Read the model definition and answer for the solid it produces. Units are mm, in the model's axes. A direction names the side the tool comes from. Round coordinates to 2 decimals unless told otherwise and drop trailing zeros. Loops run counter-clockwise (first coordinate to the right, second up) from the corner with the lowest first, then second, coordinate; pieces in that order, holes last. Notation, with made-up numbers: M 22,32 L 45,32 A20 ccw 45,57 Z; hole C -21,61.25 d10. An arc over 180 degrees is marked long. Write each question's results on one line, items separated by ' | '.
from build123d import *

# Parameters (mm, degrees)
BOSS_EXTRUDE3_DEPTH                                 = 48
SKETCH9_R                                           = 1.6
BOSS_EXTRUDE5_DEPTH                                 = 2
SKETCH6_R                                           = 1.6
BOSS_EXTRUDE6_DEPTH                                 = 2
FILLET4_R                                           = 1
FILLET5_R                                           = 12.2
CSK_FOR_M3_COUNTERSUNK_FLAT_HEAD_SCREW1_D           = 3.2
CSK_FOR_M3_COUNTERSUNK_FLAT_HEAD_SCREW1_CSINK_D     = 6.3
CSK_FOR_M3_COUNTERSUNK_FLAT_HEAD_SCREW1_CSINK_ANGLE = 90
CSK_FOR_M3_COUNTERSUNK_FLAT_HEAD_SCREW2_D           = 3.2
CSK_FOR_M3_COUNTERSUNK_FLAT_HEAD_SCREW2_CSINK_D     = 6.3
CSK_FOR_M3_COUNTERSUNK_FLAT_HEAD_SCREW2_CSINK_ANGLE = 90


with BuildPart() as part:
    # Sketch5 → Boss-Extrude3 (new, symmetric)
    with BuildSketch(Plane(origin=(0, 0, 0), x_dir=(1, 0, 0), z_dir=(0, 1, 0))):
        Polygon((0, 8.5), (0, 0), (8.5, 0), (8.5, 2), (2, 2), (2, 8.5), align=None)
    extrude(amount=BOSS_EXTRUDE3_DEPTH, both=True)

    # Sketch9 → Boss-Extrude5 (add)
    with BuildSketch(Plane.XY):
        with BuildLine():
            Line((8.5, 50), (18.5, 50))
            Line((18.5, 50), (18.5, 48.8))
            Line((18.5, 48.8), (22.7, 48.8))
            Line((22.7, 48.8), (22.7, 44))
            ThreePointArc((22.7, 44), (21.821320344, 41.878679656), (19.7, 41))
            Line((19.7, 41), (8.5, 41))
            Line((8.5, 41), (8.5, 50))
        make_face()
        with Locations((11.9, 45.8)):
            Circle(SKETCH9_R, mode=Mode.SUBTRACT)
        with Locations((19.5, 45.8)):
            Circle(SKETCH9_R, mode=Mode.SUBTRACT)
    boss_extrude5 = extrude(amount=-BOSS_EXTRUDE5_DEPTH)

    # Sketch6 → Boss-Extrude6 (add)
    with BuildSketch(Plane.ZY):
        with BuildLine():
            Line((-8.5, 41), (-19.7, 41))
            ThreePointArc((-19.7, 41), (-21.821320344, 41.878679656), (-22.7, 44))
            Line((-22.7, 44), (-22.7, 48.8))
            Line((-22.7, 48.8), (-18.5, 48.8))
            Line((-18.5, 48.8), (-18.5, 50))
            Line((-18.5, 50), (-8.5, 50))
            Line((-8.5, 50), (-8.5, 41))
        make_face()
        with Locations((-11.9, 45.8)):
            Circle(SKETCH6_R, mode=Mode.SUBTRACT)
        with Locations((-19.5, 45.8)):
            Circle(SKETCH6_R, mode=Mode.SUBTRACT)
    boss_extrude6 = extrude(amount=-BOSS_EXTRUDE6_DEPTH)

    # Mirror1: Boss-Extrude5, Boss-Extrude6 across plane
    add(boss_extrude5.mirror(Plane.ZX))
    add(boss_extrude6.mirror(Plane.ZX))

    # Fillet4
    fillet4_edges = [part.edges().sort_by_distance(p)[0] for p in [
        (0, 0, 0),
        (13.5, 50, 0),
        (0, 50, -13.5),
    ]]
    fillet(fillet4_edges, radius=FILLET4_R)

    # Fillet5
    fillet5_edges = [part.edges().sort_by_distance(p)[0] for p in [
        (8.5, -41, -1),
        (8.5, 41, -1),
        (1, 41, -8.5),
        (1, -41, -8.5),
    ]]
    fillet(fillet5_edges, radius=FILLET5_R)

    # CSK for M3 Countersunk Flat Head Screw1 (through all)
    with Locations(Plane.ZY):
        with Locations((-19.5, 45.8)):
            csk_for_m3_countersunk_flat_head_screw1 = CounterSinkHole(CSK_FOR_M3_COUNTERSUNK_FLAT_HEAD_SCREW1_D / 2, CSK_FOR_M3_COUNTERSUNK_FLAT_HEAD_SCREW1_CSINK_D / 2, counter_sink_angle=CSK_FOR_M3_COUNTERSUNK_FLAT_HEAD_SCREW1_CSINK_ANGLE)

    # CSK for M3 Countersunk Flat Head Screw2 (through all)
    with Locations(Plane.XY):
        with Locations((19.5, 45.8)):
            csk_for_m3_countersunk_flat_head_screw2 = CounterSinkHole(CSK_FOR_M3_COUNTERSUNK_FLAT_HEAD_SCREW2_D / 2, CSK_FOR_M3_COUNTERSUNK_FLAT_HEAD_SCREW2_CSINK_D / 2, counter_sink_angle=CSK_FOR_M3_COUNTERSUNK_FLAT_HEAD_SCREW2_CSINK_ANGLE)

    # Mirror2: CSK for M3 Countersunk Flat Head Screw1, CSK for M3 Countersunk Flat Head Screw2 across plane
    add(csk_for_m3_countersunk_flat_head_screw1.mirror(Plane.ZX), mode=Mode.SUBTRACT)
    add(csk_for_m3_countersunk_flat_head_screw2.mirror(Plane.ZX), mode=Mode.SUBTRACT)


solid = part.part
Item 1: The part is cut by section C-C (z = -11.9). State how many separate pieces and enclosed holes the cut face has, plus the area to 3 significant figures.
Outcome:
separate pieces: 4 | enclosed holes: 0 | area: 37.9 mm2
Item 2: Straight lines are drawn through the part: line 1 (Z direction, x = 1.8, y = -45.8); line 2 (Y direction, x = 19.5, z = -1.65); line 3 (Y direction, x = 0.6, z = -11.9). For each, find the intervals that lie inside material, in ascending order.
Outcome:
line 1: z = -22.7 to -21.1, -17.9 to -13.5, -10.3 to 0 | line 2: y = -48.8 to -47.4, -44.2 to -40.97, 40.97 to 44.2, 47.4 to 48.8 | line 3: y = -50 to -47.4, -44.2 to -37.28, 37.28 to 44.2, 47.4 to 49.92
Item 3: For faces 1 (the face through (1, -49, -8.5)), 2 (the face through (8.5, -49, -1)), 3 (the face through (2, -1, -8)), determine the directions among +Z, -Z, +X, -X, +Y, -Y from which every point of the face is accessible in a straight line to the end or side of a thin tool.
Outcome:
face 1: +Z, +X, -X, -Y | face 2: +Z, -Z, -X, -Y | face 3: -Z, +X, +Y, -Y
Item 4: The part is cut by section B-B (y = 22.5). Determine the outline of the cut face in (x, z), plus the area to 3 significant figures.
Outcome:
outline: M 0,-8.5 L 2,-8.5 L 2,-2 L 8.5,-2 L 8.5,0 L 1,0 A1 ccw 0,-1 Z | area: 29.8 mm2
Item 5: Flat-ended cylindrical pins translate along their axes: pin 1 (1 mm diameter, centred on y = 49, z = -1, fed in from -X); pin 2 (1 mm diameter, centred on x = 1.5, y = 49.5, fed in from -Z); pin 3 (5 mm diameter, centred on y = 45.8, z = -19.5, fed in from -X). Find the tip coordinate at first contact, or state that the pin passes through.
Outcome:
pin 1: stops at x = 8.5 | pin 2: stops at z = -18.5 | pin 3: stops at x = 0.65
Item 6: The mould has two halves that part along Y. Classify faces 4 (the face through (1, -48.8, -21)), 5 (the face through (0.99, 41.93, -21.87)), 6 (the face through (8.5, 49, -1)): pulls with the +Y half, pulls with the -Y half, needs draft (parallel to the pull), parting line crosses it, or undercut.
Outcome:
face 4: pulls with the -Y half | face 5: undercut | face 6: needs draft
Item 7: The part is cut by section A-A (y = 45.8). Determine the outline of the cut face in (x, z).
Outcome:
outline: M 0,-22.7 L 2,-22.7 L 2,-21.1 L 1.55,-21.1 L 0,-22.65 Z; M 0,-16.35 L 1.55,-17.9 L 2,-17.9 L 2,-13.5 L 0,-13.5 Z; M 0,-10.3 L 2,-10.3 L 2,-2 L 10.3,-2 L 10.3,0 L 1,0 A1 ccw 0,-1 Z; M 13.5,-2 L 17.9,-2 L 17.9,-1.55 L 16.35,0 L 13.5,0 Z; M 21.1,-2 L 22.7,-2 L 22.7,0 L 22.65,0 L 21.1,-1.55 Z
